Model file for the job. Use its own axes, mm. A direction names the side the tool comes from. Give positions to 0.01 mm unless a question says otherwise; leave off trailing zeros. Write each loop counter-clockwise with the first axis right and the second up, starting at its lowest first coordinate (ties: lowest second). Pieces come first, ordered by that corner, then holes.
```python
from build123d import *

# Parameters (mm, degrees)
SKETCH1_R                = 50
BOSS_EXTRUDE1_DEPTH      = 50
BOSS_EXTRUDE2_REACH      = 218.16
BOSS_EXTRUDE2_END_RADIUS = 65
SKETCH3_R                = 45


with BuildPart() as part:
    # Sketch1 → Boss-Extrude1 (new, symmetric)
    with BuildSketch(Plane.XY):
        with BuildLine():
            Line((-80, -40), (-80, 40))
            Line((-80, 40), (-23.631612274, 60.552018144))
            ThreePointArc((-23.631612274, 60.552018144), (64.978074331, 1.688151706), (-20.45553182, -61.697416623))
            Line((-20.45553182, -61.697416623), (-80, -40))
        make_face()
        Circle(SKETCH1_R, mode=Mode.SUBTRACT)
    extrude(amount=BOSS_EXTRUDE1_DEPTH, both=True)

    # Boss-Extrude2: up to this cylinder (the profile starts outside it)
    boss_extrude2_end = Plane(origin=(0, 0, 0), z_dir=(0, 0, -1)) * Cylinder(BOSS_EXTRUDE2_END_RADIUS, 567.32, mode=Mode.PRIVATE)
    # Sketch3 → Boss-Extrude2 (add, up to the surface)
    with BuildSketch(Plane.ZY.offset(-120), mode=Mode.PRIVATE) as boss_extrude2_sk1:
        with Locations(Location((0, 0, 0), (0, 0, 180))):
            Circle(SKETCH3_R)
    boss_extrude2_tool1 = extrude(boss_extrude2_sk1.sketch, amount=BOSS_EXTRUDE2_REACH, mode=Mode.PRIVATE) - boss_extrude2_end
    add(boss_extrude2_tool1.solids().sort_by_distance((120, 0, 0))[0])

    # Sketch4 → Revolve1 (revolve)
    with BuildSketch(Plane.XY, mode=Mode.PRIVATE) as revolve1_sk:
        Polygon((120, 0), (195, 0), (158.381829475, -5.301847546), (158.381829475, -13.205820305), (149, -16.667218245), (149, -25), (134, -25), (134, -20), (120, -20), align=None)
    revolve(revolve1_sk.sketch.rotate(Axis((120, 0, 0), (1, 0, 0)), 270), axis=Axis((120, 0, 0), (1, 0, 0)))


solid = part.part
```
1. Pin check, flat tips, straight feed: P1, Ø6, axis at x = 108, z = -34, coming from the +Y side; P2, Ø4, axis at x = 10.5, z = 16.5, coming from the +Y side. Stop position of each tip, or through.
Calculated:
P1: stops at y = 32.62
P2: stops at y = 64.44
2. Slice it at B-B, the plane y = 36.5. Write the cut outline in (x, z).
Calculated:
outline: (-80, -50) - (-34.17, -50) - (-34.17, 50) - (-80, 50) - close; (34.17, -50) - (53.78, -50) - (53.78, -26.32) - (120, -26.32) - (120, 26.32) - (53.78, 26.32) - (53.78, 50) - (34.17, 50) - close
3. Which spindle directions (+Z, -Z, +X, -X, +Y, -Y) get a long thin tool onto all of the face, cutting with end or side? Do faces 1 (the flat face through (-80, -1, 1)), 2 (the flat face through (158.382, 0, -6)), 3 (the cylindrical face through (126.902, 19.524, -4.336)). Say none if no direction does.
Calculated:
face 1: +Z, -Z, -X, +Y, -Y
face 2: +X
face 3: none
4. Probe probe 1 along Y at (x, z) = (0, 12); probe 2 along Y at (x, z) = (-6, -38.5); probe 3 along X at (y, z) = (-11.5, -28). List the from-to ranges inside material, lowest first.
Calculated:
probe 1: y = -65 to -50, 50 to 65
probe 2: y = -64.72 to -49.64, 49.64 to 64.72
probe 3: x = -80 to -48.66, 48.66 to 120
5. Slice it at C-C, the plane z = -38.5. Write the cut outline in (x, y), and give its area (3 significant figures).
Calculated:
outline: (-80, -40) - (-20.46, -61.7) arc R65 ccw to (60.68, -23.3) - (120, -23.3) - (120, 23.3) - (60.68, 23.3) arc R65 ccw to (-23.63, 60.55) - (-80, 40) - close; hole circle Ø100 at (0, 0)
area: 10,100 mm2
6. Slice it at D-D, the plane y = -33. Write the cut outline in (x, z).
Calculated:
outline: (-80, -50) - (-37.56, -50) - (-37.56, 50) - (-80, 50) - close; (37.56, -50) - (56, -50) - (56, -30.59) - (120, -30.59) - (120, 30.59) - (56, 30.59) - (56, 50) - (37.56, 50) - close
7. Pull direction X, two halves, no side cores. Call faces 4 (the cylindrical face through (47.69, 15.02, -0.7)), 5 (the cylindrical face through (141.395, -7.509, 23.846)), 6 (the conical face through (176.435, 2.624, -0.583)): +X half, -X half, draft (parallel to the pull), parting line (faces both ways), or undercut.
Calculated:
face 4: undercut
face 5: draft
face 6: +X half
8. Slice it at A-A, the plane x = 0. Write the cut outline in (y, z), and give its area (3 significant figures).
Calculated:
outline: (-65, -50) - (-50, -50) - (-50, 50) - (-65, 50) - close; (50, -50) - (65, -50) - (65, 50) - (50, 50) - close
area: 3,000 mm2
